Here's how the part is built. I have some questions about the finished solid (model axes, mm). A direction names the side the tool comes from. Coordinates: 2 decimals unless noted, no trailing zeros. Write each loop counter-clockwise with the first axis right and the second up, starting at its lowest first coordinate (ties: lowest second). Pieces come first, ordered by that corner, then holes. Notation, with made-up numbers: (-37, 39) -> (11, 39) arc R30 cw to (11, 71) -> close; hole circle Ø1 at (77, 65). An arc over 180 degrees is marked (long way). Put each result on its own line as item: value.
```python
from build123d import *

# Parameters (mm, degrees)
SKETCH1_W           = 13.5
SKETCH1_H           = 2
BOSS_EXTRUDE1_DEPTH = 2.2
FILLET1_R           = 0.7
SKETCH2_W           = 14.6
SKETCH2_H           = 1.9
BOSS_EXTRUDE2_DEPTH = 2.2
FILLET2_R           = 0.7
SKETCH3_W           = 11
SKETCH3_H           = 0.6
CUT_EXTRUDE1_DEPTH  = 4
SKETCH4_W           = 0.4
SKETCH4_H           = 2.5
BOSS_EXTRUDE3_DEPTH = 0.2


with BuildPart() as part:
    # Sketch1 → Boss-Extrude1 (new body)
    with BuildSketch(Plane.XY):
        Rectangle(SKETCH1_W, SKETCH1_H)
    extrude(amount=BOSS_EXTRUDE1_DEPTH)

    # Fillet1
    fillet1_edges = [part.edges().sort_by_distance(p)[0] for p in [
        (6.75, -1, 1.1),
        (-6.75, -1, 1.1),
        (-6.75, 1, 1.1),
        (6.75, 1, 1.1),
    ]]
    fillet(fillet1_edges, radius=FILLET1_R)

    # Sketch2 → Boss-Extrude2 (add)
    with BuildSketch(Plane.XY.offset(2.2)):
        Rectangle(SKETCH2_W, SKETCH2_H)
    extrude(amount=BOSS_EXTRUDE2_DEPTH)

    # Fillet2
    fillet2_edges = [part.edges().sort_by_distance(p)[0] for p in [
        (7.3, 0.95, 3.3),
        (7.3, 0, 4.4),
        (7.3, -0.95, 3.3),
        (-7.3, -0.95, 3.3),
        (-7.3, 0, 4.4),
        (-7.3, 0.95, 3.3),
    ]]
    fillet(fillet2_edges, radius=FILLET2_R)

    # Sketch3 → Cut-Extrude1 (cut)
    with BuildSketch(Plane.XY.offset(4.4)):
        with Locations((0, -0.45)):
            Rectangle(SKETCH3_W, SKETCH3_H)
    extrude(amount=-CUT_EXTRUDE1_DEPTH, mode=Mode.SUBTRACT)

    # Sketch4 → Boss-Extrude3 (add)
    with BuildSketch(Plane(origin=(0, 0, 0), x_dir=(-1, 0, 0), z_dir=(0, 0, -1))):
        with Locations((4.25, -0.25)):
            Rectangle(SKETCH4_W, SKETCH4_H)
        with Locations((3.25, -0.25)):
            Rectangle(SKETCH4_W, SKETCH4_H)
        with Locations((2.25, -0.25)):
            Rectangle(SKETCH4_W, SKETCH4_H)
        with Locations((1.25, -0.25)):
            Rectangle(SKETCH4_W, SKETCH4_H)
        with Locations((0.25, -0.25)):
            Rectangle(SKETCH4_W, SKETCH4_H)
        with Locations((-0.75, -0.25)):
            Rectangle(SKETCH4_W, SKETCH4_H)
        with Locations((-1.75, -0.25)):
            Rectangle(SKETCH4_W, SKETCH4_H)
        with Locations((-2.75, -0.25)):
            Rectangle(SKETCH4_W, SKETCH4_H)
        with Locations((-3.75, -0.25)):
            Rectangle(SKETCH4_W, SKETCH4_H)
        with Locations((3.75, 0.25)):
            Rectangle(SKETCH4_W, SKETCH4_H)
        with Locations((2.75, 0.25)):
            Rectangle(SKETCH4_W, SKETCH4_H)
        with Locations((1.75, 0.25)):
            Rectangle(SKETCH4_W, SKETCH4_H)
        with Locations((0.75, 0.25)):
            Rectangle(SKETCH4_W, SKETCH4_H)
        with Locations((-0.25, 0.25)):
            Rectangle(SKETCH4_W, SKETCH4_H)
        with Locations((-1.25, 0.25)):
            Rectangle(SKETCH4_W, SKETCH4_H)
        with Locations((-2.25, 0.25)):
            Rectangle(SKETCH4_W, SKETCH4_H)
        with Locations((-3.25, 0.25)):
            Rectangle(SKETCH4_W, SKETCH4_H)
        with Locations((-4.25, 0.25)):
            Rectangle(SKETCH4_W, SKETCH4_H)
    extrude(amount=-BOSS_EXTRUDE3_DEPTH)


solid = part.part
```
Item 1: Please list where these lines run through material, in increasing order: line 1 along Y through (x, z) = (-3.75, 2.8); line 2 along Y through (x, z) = (-1.25, 0.25); line 3 along Z through (x, y) = (5, -0.7). Write a range as from..to.
Output:
line 1: y = -0.95..-0.75, -0.15..0.95
line 2: y = -1..1
line 3: z = 0..0.4
Item 2: Imagine slicing it at C-C on y = -1.3. State how many separate pieces and enclosed holes the cut face has, then the cut area to 3 significant figures.
Output:
separate pieces: 9
enclosed holes: 0
area: 0.720 mm²
Item 3: Imagine slicing it at B-B on x = 3.25. Write out the boundary of the cut face in (y, z).
Output:
outline: (-1, 0) -> (1.5, 0) -> (1.5, 0.2) -> (1, 0.2) -> (1, 2.2) -> (0.95, 2.2) -> (0.95, 4.4) -> (-0.15, 4.4) -> (-0.15, 0.4) -> (-0.75, 0.4) -> (-0.75, 4.4) -> (-0.95, 4.4) -> (-0.95, 2.2) -> (-1, 2.2) -> close
Item 4: If we mould it in two halves opening along Y, with no side actions, what happens to faces 1 (the flat face through (0, 0, 4.4)), 2 (the flat face through (0, -0.95, 3)), 3 (the flat face through (0, -0.75, 2))? For each: released by +Y, released by -Y, zero draft, split by the parting line, or undercut.
Output:
face 1: zero draft
face 2: released by -Y
face 3: undercut
Item 5: Imagine slicing it at D-D on y = 0. Write out the boundary of the cut face in (x, z), then the cut area to 3 significant figures.
Output:
outline: (-7.3, 2.2) -> (-6.75, 2.2) -> (-6.75, 0) -> (6.75, 0) -> (6.75, 2.2) -> (7.3, 2.2) -> (7.3, 3.7) arc R0.7 ccw to (6.6, 4.4) -> (-6.6, 4.4) arc R0.7 ccw to (-7.3, 3.7) -> close
area: 61.6 mm²
Item 6: Which directions (+Z, -Z, +X, -X, +Y, -Y) give clear straight access to the entire face, cutting with the end or side of a thin tool? Please do faces 4 (the flat face through (0, 0.95, 3)), 5 (the flat face through (0, 0, 0)), 6 (the flat face through (0, -0.15, 2)).
Output:
face 4: +Z, +X, -X, +Y
face 5: -Z, +X, -X, +Y, -Y
face 6: +Z
Item 7: Imagine slicing it at A-A on z = 2.6. Write out the boundary of the cut face in (x, y).
Output:
outline: (-7.3, -0.25) arc R0.7 ccw to (-6.6, -0.95) -> (6.6, -0.95) arc R0.7 ccw to (7.3, -0.25) -> (7.3, 0.25) arc R0.7 ccw to (6.6, 0.95) -> (-6.6, 0.95) arc R0.7 ccw to (-7.3, 0.25) -> close; hole (-5.5, -0.75) -> (5.5, -0.75) -> (5.5, -0.15) -> (-5.5, -0.15) -> close
Item 8: For P1, Ø2, axis at x = 1.5, z = 2.5, coming from the +Y side, with a flat end and sliding along its axis, tell me the tip position at first contact or that it passes through.
Output:
P1: stops at y = 1
